The figure shows three views and two pictorial views of one solid part (mm, origin at its lowest corner). Answer the questions. A direction names the side the tool comes from. Coordinates: 2 decimals unless noted, no trailing zeros. Loops run counter-clockwise (first coordinate to the right, second up) from the corner with the lowest first, then second, coordinate; pieces in that order, holes last. Notation, with made-up numbers: M 0,46.5 L 21,46.5 A27 cw 21,85.5 Z; hole C 4,-16.5 d6. An arc over 180 degrees is marked long. Return JSON: item names as keys, results as strings. Group by question number.
1. Section A-A (x = 10) is taken. Write down the section's boundary in (y, z), then the cut area to 3 significant figures.
2. Section B-B (y = 15.25) is taken. Write down the section's boundary in (x, z), then the cut area to 4 significant figures.
3. Given P1, Ø1.5, axis at x = 7, z = 186.5, coming from the +Y side; P2, Ø5, axis at x = 8, z = 134.5, coming from the -Y side; P3, Ø1, axis at y = 19.5, z = 35.5, coming from the -X side; P4, Ø1, axis at x = 13, y = 3, coming from the +Z side, each flat-ended and moving along its own axis, determine where each tip first touches the part or whether it passes through.
4. Straight lines are drawn through the part: L1, parallel to Y at x = 1.75, z = 35.5; L2, parallel to Z at x = 1, y = 17.25; L3, parallel to Z at x = 1, y = 22.75 (1 decimal). For each, find the intervals that lie inside material, in ascending order. Write a range as from..to.
5. Section C-C (z = 39) is taken. Write down the section's boundary in (x, y).
6. Which of the six approach directions +Z, -Z, +X, -X, +Y, -Y give full straight-line access (tool end or side, diameter ignored) to the marked faces 1, 2 and 3?
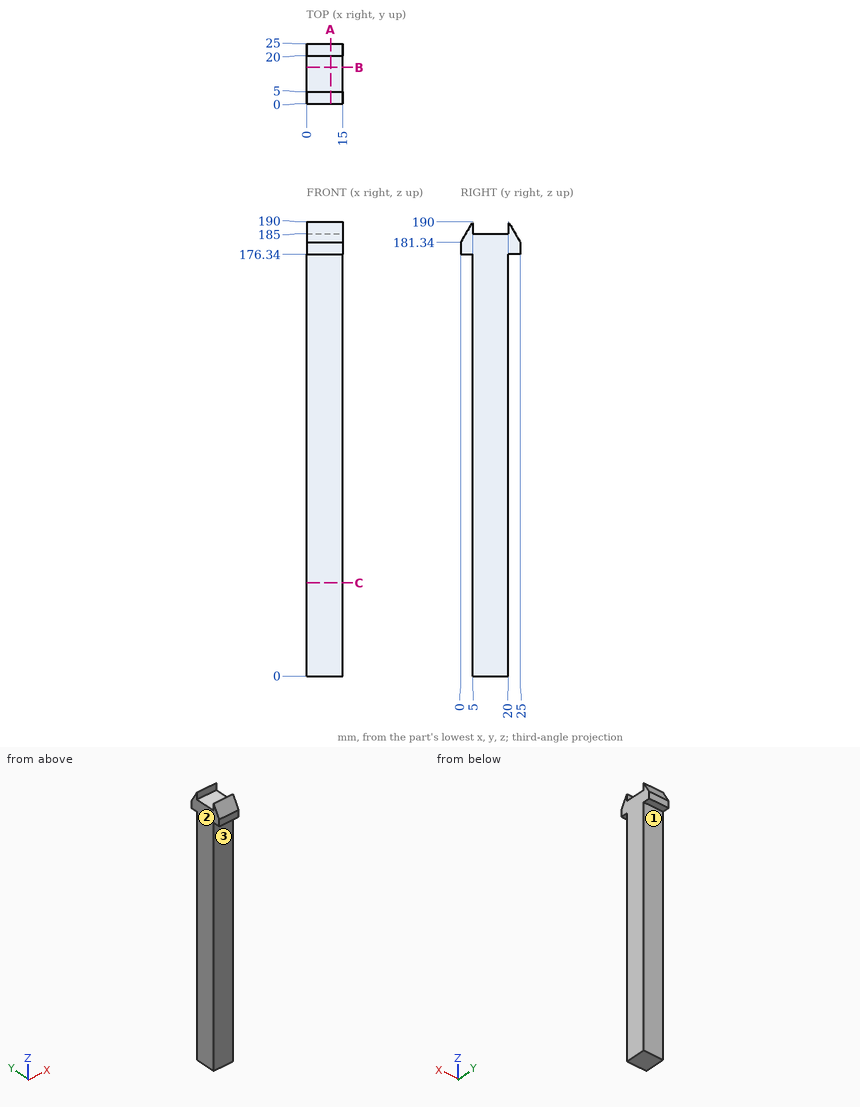
Worked out:
{
 "1": {"outline": "M 0,176.34 L 5,176.34 L 5,0 L 20,0 L 20,176.34 L 25,176.34 L 25,181.34 L 20,190 L 20,185 L 5,185 L 5,190 L 0,181.34 Z", "area": "2,870 mm^2"},
 "2": {"outline": "M 0,0 L 15,0 L 15,185 L 0,185 Z", "area": "2,775 mm^2"},
 "3": {"P1": "y = 22.45", "P2": "y = 5", "P3": "x = 0", "P4": "z = 187.4"},
 "4": {"L1": "5..20", "L2": "0..185", "L3": "176.3..185.2"},
 "5": {"outline": "M 0,5 L 15,5 L 15,20 L 0,20 Z"},
 "6": {"face 1": "-Z, +X, -X, +Y", "face 2": "+Z, -Z, -X, +Y, -Y", "face 3": "-Z, +X, -X, -Y"}
}
